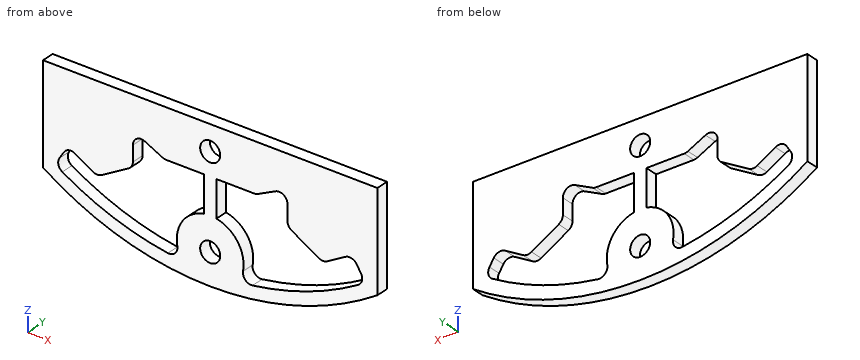
```python
from build123d import *

# Parameters (mm, degrees)
BOSS_EXTRUDE1_DEPTH  = 3
CUT_EXTRUDE12_DEPTH  = 103.574363269
SKETCH11_OUTSIDE_W   = 186.736
SKETCH11_OUTSIDE_H   = 177.534
SKETCH11_OUTSIDE_W_2 = 80
SKETCH11_OUTSIDE_H_2 = 40
CUT_EXTRUDE13_DEPTH  = 103.574363269
SKETCH12_R           = 2.4
CUT_EXTRUDE15_DEPTH  = 83.856804186
SKETCH13_W           = 3
SKETCH13_H           = 13.331578006
BOSS_EXTRUDE2_DEPTH  = 3


with BuildPart() as part:
    # Sketch1 → Boss-Extrude1 (new body)
    with BuildSketch(Plane(origin=(0, 0, 0), x_dir=(1, 0, 0), z_dir=(0, 1, 0))):
        with BuildLine():
            ThreePointArc((36.543377003, -62.616544118), (0, 72.5), (-36.543377003, -62.616544118))
            ThreePointArc((-36.543377003, -62.616544118), (-33.085954668, -63.20954405), (-30.089832649, -61.38507948))
            ThreePointArc((-30.089832649, -61.38507948), (0, -46.75), (30.089832649, -61.38507948))
            ThreePointArc((30.089832649, -61.38507948), (33.085954668, -63.20954405), (36.543377003, -62.616544118))
        make_face()
    extrude(amount=BOSS_EXTRUDE1_DEPTH)

    # Sketch10 → Cut-Extrude12 (cut, through all)
    with BuildSketch(Plane.XZ):
        with BuildLine():
            Line((-18.5, -48.031932838), (-18.5, -51.75277675))
            ThreePointArc((-18.5, -51.75277675), (-18.767949192, -52.75277675), (-19.5, -53.484827557))
            Line((-19.5, -53.484827557), (-26, -57.237604307))
            ThreePointArc((-26, -57.237604307), (-27, -57.505553499), (-28, -57.237604307))
            Line((-28, -57.237604307), (-32.336247441, -54.73407068))
            ThreePointArc((-32.336247441, -54.73407068), (-33.814934269, -54.524251533), (-35.026688711, -55.397286461))
            Line((-35.026688711, -55.397286461), (-36.057344072, -57.027343779))
            ThreePointArc((-36.057344072, -57.027343779), (-36.311279162, -58.56458095), (-35.385181403, -59.817547066))
            ThreePointArc((-35.385181403, -59.817547066), (-23.193446557, -65.515754112), (-10.132084292, -68.757478632))
            ThreePointArc((-10.132084292, -68.757478632), (-8.40348615, -68.169871795), (-7.872410817, -66.423076923))
            ThreePointArc((-7.872410817, -66.423076923), (0, -57), (7.872410817, -66.423076923))
            ThreePointArc((7.872410817, -66.423076923), (8.40348615, -68.169871795), (10.132084292, -68.757478632))
            ThreePointArc((10.132084292, -68.757478632), (23.193446557, -65.515754112), (35.385181403, -59.817547066))
            ThreePointArc((35.385181403, -59.817547066), (36.311279162, -58.56458095), (36.057344072, -57.027343779))
            Line((36.057344072, -57.027343779), (35.026688711, -55.397286461))
            ThreePointArc((35.026688711, -55.397286461), (33.814934269, -54.524251533), (32.336247441, -54.73407068))
            Line((32.336247441, -54.73407068), (28, -57.237604307))
            ThreePointArc((28, -57.237604307), (27, -57.505553499), (26, -57.237604307))
            Line((26, -57.237604307), (19.5, -53.484827557))
            ThreePointArc((19.5, -53.484827557), (18.767949192, -52.75277675), (18.5, -51.75277675))
            Line((18.5, -51.75277675), (18.5, -48.031932838))
            ThreePointArc((18.5, -48.031932838), (17.558247208, -46.334843316), (15.619887154, -46.235992589))
            Line((15.619887154, -46.235992589), (11.416400149, -48.295940249))
            ThreePointArc((11.416400149, -48.295940249), (10.988017035, -48.448317287), (10.536287302, -48.5))
            Line((10.536287302, -48.5), (-10.536287302, -48.5))
            ThreePointArc((-10.536287302, -48.5), (-10.988017035, -48.448317287), (-11.416400149, -48.295940249))
            Line((-11.416400149, -48.295940249), (-15.619887154, -46.235992589))
            ThreePointArc((-15.619887154, -46.235992589), (-17.558247208, -46.334843316), (-18.5, -48.031932838))
        make_face()
    extrude(amount=-CUT_EXTRUDE12_DEPTH, mode=Mode.SUBTRACT)

    # Sketch11 outside → Cut-Extrude13 (cut, through all)
    with BuildSketch(Plane.XZ):
        with Locations((0, -4.601)):
            Rectangle(SKETCH11_OUTSIDE_W, SKETCH11_OUTSIDE_H)
        with Locations((0, -57)):
            Rectangle(SKETCH11_OUTSIDE_W_2, SKETCH11_OUTSIDE_H_2, mode=Mode.SUBTRACT)
    extrude(amount=-CUT_EXTRUDE13_DEPTH, mode=Mode.SUBTRACT)

    # Sketch12 → Cut-Extrude15 (cut, through all)
    with BuildSketch(Plane.XZ):
        with Locations(Location((0, -65, 0), (0, 0, 270))):
            Circle(SKETCH12_R)
        with Locations(Location((0, -43, 0), (0, 0, 270))):
            Circle(SKETCH12_R)
    extrude(amount=-CUT_EXTRUDE15_DEPTH, mode=Mode.SUBTRACT)

    # Sketch13 → Boss-Extrude2 (add)
    with BuildSketch(Plane.XZ):
        with Locations((0, -53.718139369)):
            Rectangle(SKETCH13_W, SKETCH13_H)
    extrude(amount=-BOSS_EXTRUDE2_DEPTH)


solid = part.part
```
The listing builds one solid part. Answer for the finished solid, in the listing's coordinates (mm). Give positions to 0.01 mm unless a question says otherwise; leave off trailing zeros. Write each loop counter-clockwise with the first axis right and the second up, starting at its lowest first coordinate (ties: lowest second). Pieces come first, ordered by that corner, then holes. Notation, with made-up numbers: (38, 76) -> (62, 76) arc R21 ccw to (62, 80) -> close; hole circle Ø9 at (36.5, 2). An arc over 180 degrees is marked (long way). Use one line per item in the form item = value.
1) Each of these flat-tipped pins is pushed along its axis until it touches: P1, Ø3, axis at x = 0, z = -43, coming from the +Y side; P2, Ø1.5, axis at x = -6.5, y = 2, coming from the -Z side; P3, Ø1.5, axis at x = 4.5, y = 2, coming from the -Z side. Where does it stop, or does it pass through?
Result:
P1 = through
P2 = -72.27
P3 = -72.4
2) Section B-B on x = 0 is taken. Write down the section's boundary in (y, z).
Result:
outline = (0, -72.5) -> (3, -72.5) -> (3, -67.4) -> (0, -67.4) -> close; (0, -62.6) -> (3, -62.6) -> (3, -45.4) -> (0, -45.4) -> close; (0, -40.6) -> (3, -40.6) -> (3, -37) -> (0, -37) -> close
3) Section D-D on z = -52.5 is taken. Write down the section's boundary in (x, y).
Result:
outline = (-40, 0) -> (-18.64, 0) -> (-18.64, 3) -> (-40, 3) -> close; (-1.5, 0) -> (1.5, 0) -> (1.5, 3) -> (-1.5, 3) -> close; (18.64, 0) -> (40, 0) -> (40, 3) -> (18.64, 3) -> close
4) Straight lines are drawn through the part: probe 1 along X at (y, z) = (2.45, -50.5); probe 2 along X at (y, z) = (2.2, -43); probe 3 along X at (y, z) = (0.5, -45). For each, find the intervals that lie inside material, in ascending order.
Result:
probe_1 = -40 to -18.5, -1.5 to 1.5, 18.5 to 40
probe_2 = -40 to -2.4, 2.4 to 40
probe_3 = -40 to -1.33, 1.33 to 40
5) Section C-C on x = -24 is taken. Write down the section's boundary in (y, z), plus the area to 3 significant figures.
Result:
outline = (0, -68.41) -> (3, -68.41) -> (3, -65.22) -> (0, -65.22) -> close; (0, -56.08) -> (3, -56.08) -> (3, -37) -> (0, -37) -> close
area = 66.8 mm²
6) Section A-A on z = -43 is taken. Write down the section's boundary in (x, y).
Result:
outline = (-40, 0) -> (-2.4, 0) -> (-2.4, 3) -> (-40, 3) -> close; (2.4, 0) -> (40, 0) -> (40, 3) -> (2.4, 3) -> close
